from build123d import *

# Parameters (mm, degrees)
SKETCH1_W           = 296
SKETCH1_H           = 182
SKETCH1_R           = 1.5
BOSS_EXTRUDE1_DEPTH = 12
SKETCH2_R           = 1.5
CUT_EXTRUDE1_DEPTH  = 20
CUT_EXTRUDE2_START  = 276
SKETCH2_2_R         = 1.5
CUT_EXTRUDE2_DEPTH  = 20
CUT_EXTRUDE4_START  = -182
SKETCH5_R           = 1.5
CUT_EXTRUDE4_DEPTH  = 10
CUT_EXTRUDE5_START  = -10
SKETCH5_3_R         = 1.5
CUT_EXTRUDE5_DEPTH  = 10
SKETCH7_W           = 25
SKETCH7_H           = 12
CUT_EXTRUDE6_DEPTH  = 1
CUT_EXTRUDE7_START  = -182
SKETCH7_2_W         = 25
SKETCH7_2_H         = 12
CUT_EXTRUDE7_DEPTH  = 1


with BuildPart() as part:
    # Sketch1 → Boss-Extrude1 (new body)
    with BuildSketch(Plane(origin=(0, 0, 0), x_dir=(1, 0, 0), z_dir=(0, 1, 0))):
        with Locations((148, 91)):
            Rectangle(SKETCH1_W, SKETCH1_H)
        with Locations(Location((188, 160, 0), (0, 0, 270))):
            Circle(SKETCH1_R, mode=Mode.SUBTRACT)
    extrude(amount=BOSS_EXTRUDE1_DEPTH)

    # Sketch2 → Cut-Extrude1 (cut)
    with BuildSketch(Plane(origin=(0, 0, 0), x_dir=(0, 0, -1), z_dir=(1, 0, 0))):
        with Locations((162, 6)):
            Circle(SKETCH2_R)
        with Locations((34, 6)):
            Circle(SKETCH2_R)
    extrude(amount=CUT_EXTRUDE1_DEPTH, mode=Mode.SUBTRACT)

    # Sketch2<2> → Cut-Extrude2 (cut)
    with BuildSketch(Plane(origin=(0, 0, 0), x_dir=(0, 0, -1), z_dir=(1, 0, 0)).offset(CUT_EXTRUDE2_START)):
        with Locations((162, 6)):
            Circle(SKETCH2_2_R)
        with Locations((34, 6)):
            Circle(SKETCH2_2_R)
    extrude(amount=CUT_EXTRUDE2_DEPTH, mode=Mode.SUBTRACT)

    # Cut-Extrude3 cone 1 section (through the dimple's axis) → Cut-Extrude3 (revolve, cut)
    with BuildSketch(Plane(origin=(188, 12, -160), x_dir=(0, 0, 1), z_dir=(1, 0, 0))):
        Polygon((0, 0), (3, 0), (0, 3), align=None)
    revolve(axis=Axis((188, 12, -160), (0, -1, 0)), mode=Mode.SUBTRACT)

    # Sketch5 → Cut-Extrude4 (cut)
    with BuildSketch(Plane.XY.offset(CUT_EXTRUDE4_START)):
        with Locations((21, 6)):
            Circle(SKETCH5_R)
        with Locations((34, 6)):
            Circle(SKETCH5_R)
        with Locations((275, 6)):
            Circle(SKETCH5_R)
        with Locations((262, 6)):
            Circle(SKETCH5_R)
    extrude(amount=CUT_EXTRUDE4_DEPTH, mode=Mode.SUBTRACT)

    # Sketch5<3> → Cut-Extrude5 (cut)
    with BuildSketch(Plane.XY.offset(CUT_EXTRUDE5_START)):
        with Locations((21, 6)):
            Circle(SKETCH5_3_R)
        with Locations((34, 6)):
            Circle(SKETCH5_3_R)
        with Locations((275, 6)):
            Circle(SKETCH5_3_R)
        with Locations((262, 6)):
            Circle(SKETCH5_3_R)
    extrude(amount=CUT_EXTRUDE5_DEPTH, mode=Mode.SUBTRACT)

    # Sketch7 → Cut-Extrude6 (cut)
    with BuildSketch(Plane.XY):
        with Locations((27.5, 6)):
            Rectangle(SKETCH7_W, SKETCH7_H)
        with Locations((268.5, 6)):
            Rectangle(SKETCH7_W, SKETCH7_H)
    extrude(amount=-CUT_EXTRUDE6_DEPTH, mode=Mode.SUBTRACT)

    # Sketch7<2> → Cut-Extrude7 (cut)
    with BuildSketch(Plane.XY.offset(CUT_EXTRUDE7_START)):
        with Locations((27.5, 6)):
            Rectangle(SKETCH7_2_W, SKETCH7_2_H)
        with Locations((268.5, 6)):
            Rectangle(SKETCH7_2_W, SKETCH7_2_H)
    extrude(amount=CUT_EXTRUDE7_DEPTH, mode=Mode.SUBTRACT)


solid = part.part
Read the model definition and answer for the solid it produces. Units are mm, in the model's axes. A direction names the side the tool comes from. Give positions to 0.01 mm unless a question says otherwise; leave off trailing zeros. Answer in a Markdown table with one row per item. Add a question column.
Item 1: Find the intervals of material crossed by L1, parallel to X at y = 6, z = -3.75; L2, parallel to Y at x = 34, z = -2.75; L3, parallel to Z at x = 263.5, y = 10, in increasing order.
Item 2: A tool of negligible diameter and unlimited length cuts with its end or side. For faces 1 (the face through (268, 6, -181)), 2 (the face through (27, 6, -1)), 3 (the face through (146, 0, -92)), from which of +Z, -Z, +X, -X, +Y, -Y can it reach the whole face along a straight path? Write none if from no direction.
Item 3: Flat-ended cylindrical pins translate along their axes: P1, Ø0.9, axis at x = 262.5, y = 6.5, coming from the +Z side; P2, Ø2.5, axis at y = 6, z = -162, coming from the +X side; P3, Ø2.5, axis at x = 188, z = -160, coming from the +Y side; P4, Ø2.5, axis at x = 21.5, y = 6.5, coming from the +Z side. Find the tip coordinate at first contact, or state that the pin passes through.
Item 4: Determine the mould class of faces 4 (the face through (0, 6, -90)), 5 (the face through (296, 6, -90)), 6 (the face through (288, 6, 0)), 7 (the face through (186, 11, -160)) for opening direction X: pulls with the +X half, pulls with the -X half, needs draft (parallel to the pull), parting line crosses it, or undercut.
Recorded:
| question | item | result |
|---|---|---|
| 1 | L1 | x = 0 to 19.5, 22.5 to 32.5, 35.5 to 260.5, 263.5 to 273.5, 276.5 to 296 |
| 1 | L2 | y = 0 to 4.5, 7.5 to 12 |
| 1 | L3 | z = -181 to -1 |
| 2 | face 1 | -Z, +Y, -Y |
| 2 | face 2 | +Z, +Y, -Y |
| 2 | face 3 | +Z, -Z, +X, -X, -Y |
| 3 | P1 | stops at z = -10 |
| 3 | P2 | stops at x = 276 |
| 3 | P3 | passes through |
| 3 | P4 | stops at z = -1 |
| 4 | face 4 | pulls with the -X half |
| 4 | face 5 | pulls with the +X half |
| 4 | face 6 | needs draft |
| 4 | face 7 | undercut |
